Can you work these out from the model? Positions are in its coordinate system, mm. Give positions to 0.01 mm unless a question says otherwise; leave off trailing zeros. Order: outer loops, then holes, each group sorted by start corner. A loop starts at its lowest first (then second) coordinate and runs counter-clockwise, first axis right, second up.
```python
from build123d import *

# Parameters (mm, degrees)
SKETCH_1_R      = 1.5
SKETCH_1_W      = 10
SKETCH_1_H      = 3
EXTRUDE_1_DEPTH = 3.175


with BuildPart() as part:
    # 草图1 → 凸台-拉伸1 (new body)
    with BuildSketch(Plane(origin=(0, 0, 0), x_dir=(1, 0, 0), z_dir=(0, 1, 0))):
        with BuildLine():
            Line((-25, -10), (-95.916630466, -10))
            ThreePointArc((-95.916630466, -10), (-112.922283606, 11.016502751), (-125.39936204, 35))
            Line((-125.39936204, 35), (-136.106575888, 35))
            ThreePointArc((-136.106575888, 35), (-121.687593109, 6.15122269), (-101.248422592, -18.796709594))
            add(Edge.make_bspline(
                [(-101.248422592, -18.796709594), (0, -21.367886927), (101.248422592, -18.796709594)],
                knots=[1.075169889, 1.075169889, 1.075169889, 2.066422765, 2.066422765, 2.066422765], degree=2, weights=[1, 0.879670959, 1]))
            ThreePointArc((101.248422592, -18.796709594), (121.687593109, 6.15122269), (136.106575888, 35))
            Line((136.106575888, 35), (125.39936204, 35))
            ThreePointArc((125.39936204, 35), (112.922283606, 11.016502751), (95.916630466, -10))
            Line((95.916630466, -10), (25, -10))
            Line((25, -10), (25, 0))
            ThreePointArc((25, 0), (23.535533906, 3.535533906), (20, 5))
            Line((20, 5), (-20, 5))
            ThreePointArc((-20, 5), (-23.535533906, 3.535533906), (-25, 0))
            Line((-25, 0), (-25, -10))
        make_face()
        with Locations((-20, 0)):
            Circle(SKETCH_1_R, mode=Mode.SUBTRACT)
        with Locations((20, 0)):
            Circle(SKETCH_1_R, mode=Mode.SUBTRACT)
        with Locations((0, -6)):
            Rectangle(SKETCH_1_W, SKETCH_1_H, mode=Mode.SUBTRACT)
    extrude(amount=EXTRUDE_1_DEPTH)


solid = part.part
```
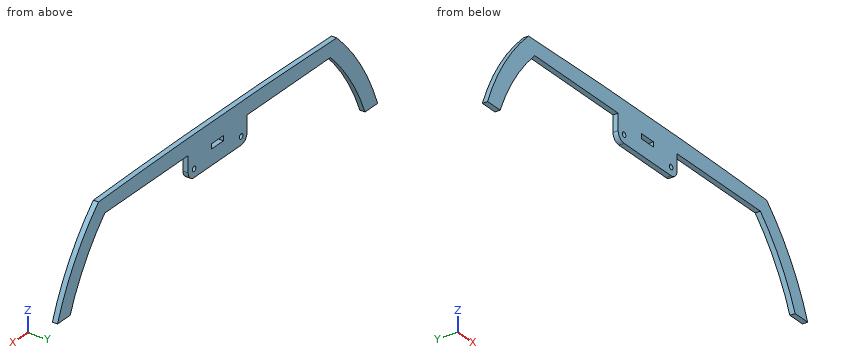
1) I'm going to push flat-ended pins straight in: pin 1 Ø5 at (x, z) = (20, 0) entering from +Y (3 decimals); pin 2 Ø1 at (y, z) = (1.5, 4.5) entering from +X; pin 3 Ø1.5 at (y, z) = (2, 6) entering from -X; pin 4 Ø1.6 at (x, y) = (1, 1.5) entering from -Z. Where does each tip first touch, or does it pass through?
2) Suppose I cut it at C-C (z = -29.5). Please give me the cut outline in (x, y) (3 decimals).
3) Suppose I cut it at A-A (z = -13.5). Please give me the cut outline in (x, y) (3 decimals).
4) Suppose I cut it at B-B (y = 2.3). Give the number of separate pieces and of enclosed holes in the cut face, and give its area (3 significant figures).
5) If I drill on line 1 (Z direction, x = -20, y = 1.3); line 2 (X direction, y = 0.8, z = 2); line 3 (X direction, y = 1.8, z = 0), over which ranges is the centre line in solid material (lowest first)?
Results:
1. pin 1: stops at y = 3.175
1. pin 2: stops at x = 114.47
1. pin 3: stops at x = -113.49
1. pin 4: stops at z = -5
2. outline: (-133.958, 0) - (-123.064, 0) - (-123.064, 3.175) - (-133.958, 3.175) - close; (123.064, 0) - (133.958, 0) - (133.958, 3.175) - (123.064, 3.175) - close
3. outline: (-126.146, 0) - (-114.511, 0) - (-114.511, 3.175) - (-126.146, 3.175) - close; (114.511, 0) - (126.146, 0) - (126.146, 3.175) - (114.511, 3.175) - close
4. separate pieces: 1
4. enclosed holes: 3
4. area: 3,780 mm2
5. line 1: z = -5 to -1.5, 1.5 to 19.96
5. line 2: x = -116 to -103.23, -25 to 25, 103.23 to 116
5. line 3: x = -117.47 to -104.88, -25 to -21.5, -18.5 to 18.5, 21.5 to 25, 104.88 to 117.47
